```python
from build123d import *

# Parameters (mm, degrees)
SKETCH1_W           = 60
SKETCH1_H           = 60
BOSS_EXTRUDE1_DEPTH = 40
FILLET1_R           = 3
FILLET2_R           = 3
SKETCH2_R           = 20
CUT_EXTRUDE1_DEPTH  = 1


with BuildPart() as part:
    # Sketch1 → Boss-Extrude1 (new body)
    with BuildSketch(Plane.XY):
        with Locations((5, -3.4375)):
            Rectangle(SKETCH1_W, SKETCH1_H)
    extrude(amount=BOSS_EXTRUDE1_DEPTH)

    # Fillet1
    fillet1_edges = [part.edges().sort_by_distance(p)[0] for p in [
        (-25, 26.5625, 20),
        (35, 26.5625, 20),
        (35, -33.4375, 20),
        (-25, -33.4375, 20),
    ]]
    fillet(fillet1_edges, radius=FILLET1_R)

    # Fillet2
    fillet2_edges = [part.edges().sort_by_distance(p)[0] for p in [
        (35, -3.4375, 0),
        (-25, -3.4375, 0),
        (5, 26.5625, 0),
        (5, -33.4375, 0),
        (34.121320344, 25.683820344, 0),
        (-24.121320344, 25.683820344, 0),
        (-24.121320344, -32.558820344, 0),
        (34.121320344, -32.558820344, 0),
    ]]
    fillet(fillet2_edges, radius=FILLET2_R)

    # Sketch2 → Cut-Extrude1 (cut)
    with BuildSketch(Plane(origin=(0, 0, 0), x_dir=(-1, 0, 0), z_dir=(0, 0, -1))):
        with Locations((-5, -3.4375)):
            Circle(SKETCH2_R)
    extrude(amount=-CUT_EXTRUDE1_DEPTH, mode=Mode.SUBTRACT)


solid = part.part
```
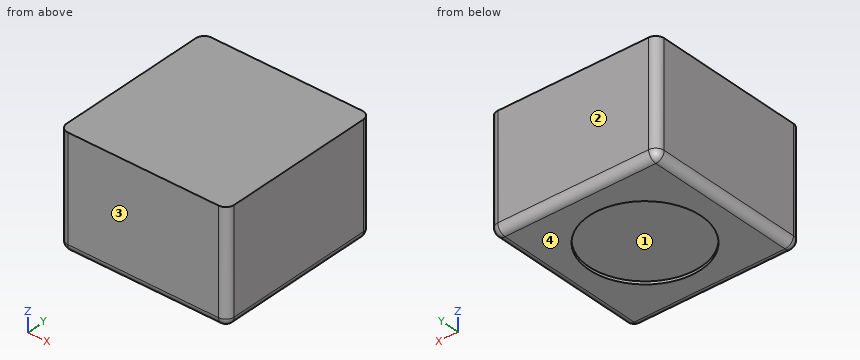
Design review of the part built by this model. Coordinates are the model's own, in mm. Face numbers are marked on the shaded views. Give positions to 0.01 mm unless a question says otherwise; leave off trailing zeros. Loops run counter-clockwise (first coordinate to the right, second up) from the corner with the lowest first, then second, coordinate; pieces in that order, holes last. Notation, with made-up numbers: M -32,-37.5 L -6,-37.5 A23 ccw -6,-5.5 Z; hole C -10,27 d10. An arc over 180 degrees is marked long. Return JSON: item names as keys, results as strings. Group by question number.
Item 1: Mouldability with a two-part tool opening along Y and no side actions: class the marked faces 1, 2, 3 and 4 as released by +Y, released by -Y, zero draft, split by the parting line, or undercut.
Item 2: We need section B-B (y = 0). Give the boundary of the cut face in (x, z).
Item 3: For probe 1 along Y at (x, z) = (5, 0.85); probe 2 along Z at (x, y) = (22.5, 0.5); probe 3 along Y at (x, z) = (5, 0.75), list the stretches that pass through material, from the lowest coordinate up.
Item 4: We need section A-A (x = 5). Give the boundary of the cut face in (y, z), and give its area (3 significant figures).
Item 5: Insertion check: pin 1 Ø20 at (x, y) = (5.5, -10) entering from -Z. The pin has a flat end and moves straight along its axis. Give the tip position at first contact, or say it passes through.
Output:
{
 "1": {"face 1": "undercut", "face 2": "released by +Y", "face 3": "released by -Y", "face 4": "zero draft"},
 "2": {"outline": "M -25,3 A3 ccw -22,0 L -14.7,0 L -14.7,1 L 24.7,1 L 24.7,0 L 32,0 A3 ccw 35,3 L 35,40 L -25,40 Z"},
 "3": {"probe 1": "y = -32.53 to -23.44, 16.56 to 25.65", "probe 2": "z = 1 to 40", "probe 3": "y = -32.42 to -23.44, 16.56 to 25.55"},
 "4": {"outline": "M -33.44,3 A3 ccw -30.44,0 L -23.44,0 L -23.44,1 L 16.56,1 L 16.56,0 L 23.56,0 A3 ccw 26.56,3 L 26.56,40 L -33.44,40 Z", "area": "2,360 mm^2"},
 "5": {"pin 1": "stops at z = 1"}
}
